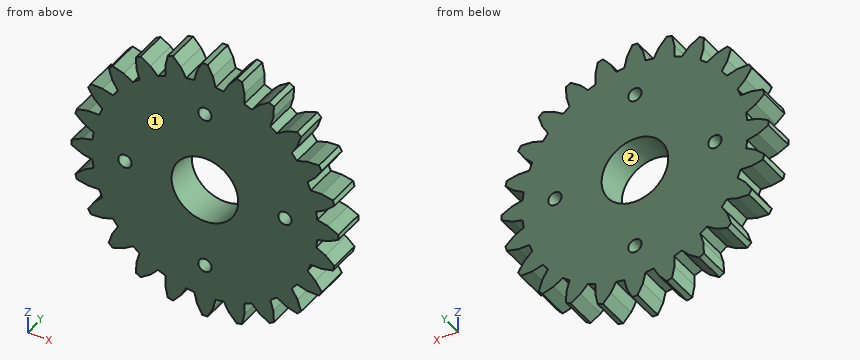
```python
from build123d import *

# Parameters (mm, degrees)
BOSS_EXTRUDE1_DEPTH = 5
SKETCH4_R           = 5
CUT_EXTRUDE1_DEPTH  = 5
SKETCH5_R           = 1
CUT_EXTRUDE2_DEPTH  = 5


with BuildPart() as part:
    # Sketch2 → Boss-Extrude1 (new body)
    with BuildSketch(Plane(origin=(0, 0, 0), x_dir=(1, 0, 0), z_dir=(0, 1, 0))):
        Polygon((62.172127475, 64.438287146), (63.746631591, 64.052516421), (65.320772998, 63.251970245), (65.320772998, 62.437646696), (63.746631591, 61.63710052), (62.172127475, 61.251330223), (62.010422663, 60.022472316), (63.431319755, 59.242350893), (64.744655445, 58.061714434), (64.533883435, 57.275066391), (62.806134576, 56.909358138), (61.185584837, 56.944164493), (60.711227056, 55.799059379), (61.881832707, 54.677762874), (62.844929445, 53.197526256), (62.437646696, 52.492214089), (60.674124543, 52.585997689), (59.117748594, 53.03908454), (58.363248469, 52.055804998), (59.203797973, 50.66971469), (59.750789184, 48.990670319), (59.174913579, 48.414794286), (57.495869208, 48.961785926), (56.1097789, 49.80233543), (55.126499358, 49.047834876), (55.579586209, 47.491459356), (55.67336981, 45.727937202), (54.968057642, 45.320654453), (53.487820596, 46.283751191), (52.366524519, 47.454356415), (51.221419405, 46.979999061), (51.25622576, 45.359448894), (50.890517507, 43.631700463), (50.103869465, 43.420928454), (48.923233005, 44.734264143), (48.143111582, 46.155161235), (46.914253675, 45.993456423), (46.528483378, 44.418952307), (45.727937202, 42.8448109), (44.913613653, 42.8448109), (44.113067477, 44.418952307), (43.727296752, 45.993456423), (42.498439273, 46.155161235), (41.718317422, 44.734264143), (40.537680963, 43.420928454), (39.751033348, 43.631700463), (39.385325095, 45.359448894), (39.420131451, 46.979999061), (38.275026336, 47.454356415), (37.153729831, 46.283751191), (35.673492785, 45.320654453), (34.968181046, 45.727937202), (35.061964647, 47.491459356), (35.515051497, 49.047834876), (34.531771955, 49.80233543), (33.145681219, 48.961785926), (31.466637276, 48.414794286), (30.890761243, 48.990670319), (31.437752883, 50.66971469), (32.278302387, 52.055804998), (31.523801833, 53.03908454), (29.967425885, 52.585997689), (28.20390416, 52.492214089), (27.796621411, 53.197526256), (28.759718149, 54.677762874), (29.930323372, 55.799059379), (29.455966018, 56.944164493), (27.835415852, 56.909358138), (26.107666992, 57.275066391), (25.896895411, 58.061714434), (27.210231101, 59.242350893), (28.631127764, 60.022472316), (28.46942338, 61.251330223), (26.894919264, 61.63710052), (25.320777429, 62.437646696), (25.320777429, 63.251970245), (26.894919264, 64.052516421), (28.46942338, 64.438287146), (28.631127764, 65.667144625), (27.210231101, 66.447266476), (25.896895411, 67.627902507), (26.107666992, 68.41455055), (27.835415852, 68.780258803), (29.455966018, 68.745452448), (29.930323372, 69.890557562), (28.759718149, 71.011854067), (27.796621411, 72.492090685), (28.20390416, 73.197402852), (29.967425885, 73.103619252), (31.523801833, 72.650532401), (32.278302387, 73.633811943), (31.437752883, 75.019902251), (30.890761243, 76.698946622), (31.466637276, 77.274822655), (33.145681219, 76.727831015), (34.531771955, 75.887281511), (35.515051497, 76.641782065), (35.061964647, 78.198157585), (34.968181046, 79.961679739), (35.673492785, 80.368962487), (37.153729831, 79.40586575), (38.275026336, 78.235260526), (39.420131451, 78.70961788), (39.385325095, 80.330168047), (39.751033348, 82.057916906), (40.537680963, 82.268688487), (41.718317422, 80.955352798), (42.498439273, 79.534456134), (43.727296752, 79.696160518), (44.113067477, 81.270664634), (44.913613653, 82.844806041), (45.727937202, 82.844806041), (46.528483378, 81.270664634), (46.914253675, 79.696160518), (48.143111582, 79.534456134), (48.923233005, 80.955352798), (50.103869465, 82.268688487), (50.890517507, 82.057916906), (51.25622576, 80.330168047), (51.221419405, 78.70961788), (52.366524519, 78.235260526), (53.487820596, 79.40586575), (54.968057642, 80.368962487), (55.67336981, 79.961679739), (55.579586209, 78.198157585), (55.126499358, 76.641782065), (56.1097789, 75.887281511), (57.495869208, 76.727831015), (59.174913579, 77.274822655), (59.750789184, 76.698946622), (59.203797973, 75.019902251), (58.363248469, 73.633811943), (59.117748594, 72.650532401), (60.674124543, 73.103619252), (62.437646696, 73.197402852), (62.844929445, 72.492090685), (61.881832707, 71.011854067), (60.711227056, 69.890557562), (61.185584837, 68.745452448), (62.806134576, 68.780258803), (64.533883435, 68.41455055), (64.744655445, 67.627902507), (63.431319755, 66.447266476), (62.010422663, 65.667144625), align=None)
    extrude(amount=BOSS_EXTRUDE1_DEPTH)

    # Sketch4 → Cut-Extrude1 (cut)
    with BuildSketch(Plane(origin=(0, 0, 0), x_dir=(1, 0, 0), z_dir=(0, 1, 0))):
        with Locations((45.320775214, 62.84480847)):
            Circle(SKETCH4_R)
    extrude(amount=CUT_EXTRUDE1_DEPTH, mode=Mode.SUBTRACT)

    # Sketch5 → Cut-Extrude2 (cut)
    with BuildSketch(Plane(origin=(0, 0, 0), x_dir=(1, 0, 0), z_dir=(0, 1, 0))):
        with Locations((45.320775428, 50.84480847)):
            Circle(SKETCH5_R)
        with Locations((33.320775428, 62.84480847)):
            Circle(SKETCH5_R)
        with Locations((45.320775428, 74.84480847)):
            Circle(SKETCH5_R)
        with Locations((57.320775428, 62.84480847)):
            Circle(SKETCH5_R)
    extrude(amount=CUT_EXTRUDE2_DEPTH, mode=Mode.SUBTRACT)


solid = part.part
```
Model file for the job. Use its own axes, mm. Face numbers are marked on the shaded views. Give positions to 0.01 mm unless a question says otherwise; leave off trailing zeros. Write each loop counter-clockwise with the first axis right and the second up, starting at its lowest first coordinate (ties: lowest second). Pieces come first, ordered by that corner, then holes. Notation, with made-up numbers: (68.25, 8.25) - (94.25, 8.25) arc R12 ccw to (94.25, 23.25) - close; hole circle Ø8 at (87.5, 31.5). An arc over 180 degrees is marked (long way). One line per question, with ' | ' between items. Start each with the question number.
(1) Slice it at C-C on z = -70.5. Write the cut outline in (x, y).
(2) Two-plate mould, pull along X, no slides. Class the marked faces 1 and 2: +X half, -X half, draft (parallel to the pull), parting line (faces both ways), or undercut.
(3) Pin check, flat tips, straight feed: P1, Ø1.6, axis at x = 45.32, z = -74.84, coming from the +Y side; P2, Ø1.5, axis at x = 56.5, y = 2, coming from the -Z side; P3, Ø1, axis at y = 2.5, z = -60, coming from the -X side; P4, Ø2, axis at x = 37, y = 2.5, coming from the +Z side. Stop position of each tip, or through.
(4) Slice it at B-B on y = 4.1. Give the number of separate pieces and of enclosed holes in the cut face, plus the area to 3 significant figures.
(5) Slice it at A-A on z = -54. Write the cut outline in (x, y).
(6) Wall check: line 1 along X through (y, z) = (3.3, -63); line 2 along Z through (x, y) = (31.5, 4.15); line 3 along X through (y, z) = (3.5, -81). Give the ranges that are in metal, low to high. Write a range as from..to.
Results below:
1) outline: (29.29, 0) - (61.35, 0) - (61.35, 5) - (29.29, 5) - close
2) face 1: draft | face 2: undercut
3) P1: through | P2: z = -76.58 | P3: x = 27.68 | P4: z = -45.53
4) separate pieces: 1 | enclosed holes: 5 | area: 972 mm^2
5) outline: (28.32, 0) - (62.32, 0) - (62.32, 5) - (28.32, 5) - close
6) line 1: 25.32..32.33, 34.31..40.32, 50.32..56.33, 58.31..65.32 | line 2: -77.26..-74.92, -72.66..-53.03, -50.77..-48.43 | line 3: 39.53..41.68, 44.05..46.59, 48.96..51.11
